```python
from build123d import *

# Parameters (mm, degrees)
F4_DEPTH = 2.3876
F5_SIZE2 = 0.762
F5_SIZE  = 0.762


with BuildPart() as f1:
    # F0 (on Right) → F1 (revolve)
    with BuildSketch(Plane.YZ):
        with BuildLine():
            ThreePointArc((-5.5626, 9.525), (-6.7410456972, 4.8271528886), (-7.1374, 0))
            Line((-7.1374, 0), (7.1374, 0))
            Line((7.1374, 0), (7.1374, 3.175))
            Line((7.1374, 3.175), (-2.3622, 3.175))
            Line((-2.3622, 3.175), (-2.3622, 9.525))
            Line((-2.3622, 9.525), (-5.5626, 9.525))
        make_face()
    revolve(axis=Axis((0, 0, 0), (0, 1, 0)))

    # F3 (on offset) → F4 (cut)
    with BuildSketch(Plane.XZ.offset(7.1374)):
        with BuildLine():
            Line((9.4923983397, 0.7874), (-9.4923983397, 0.7874))
            ThreePointArc((-9.4923983397, 0.7874), (-9.525, 0), (-9.4923983397, -0.7874))
            Line((-9.4923983397, -0.7874), (9.4923983397, -0.7874))
            ThreePointArc((9.4923983397, -0.7874), (9.525, 0), (9.4923983397, 0.7874))
        make_face()
    extrude(amount=-F4_DEPTH, mode=Mode.SUBTRACT)

    # F5
    f5_edges = [f1.edges().sort_by_distance(p)[0] for p in [
        (0, 7.1374, -3.175),
    ]]
    chamfer(f5_edges, length=F5_SIZE, length2=F5_SIZE2)


solid = f1.part
```
Source: CAD feature listing. Evaluate the final solid. Frame: model axes, mm. A direction names the side the tool comes from. Give positions to 0.01 mm unless a question says otherwise; leave off trailing zeros. Write each loop counter-clockwise with the first axis right and the second up, starting at its lowest first coordinate (ties: lowest second). Pieces come first, ordered by that corner, then holes. Notation, with made-up numbers: (69.5, -19.75) - (91.5, -19.75) arc R24 ccw to (91.5, -0.75) - close; hole circle Ø7 at (77, 8.5). An arc over 180 degrees is marked (long way). One line per item, written item: value. Start each with the question number.
Q1. Material intervals for probe 1 along Z at (x, y) = (5.5, -5); probe 2 along Z at (x, y) = (-7.75, -5.5); probe 3 along Y at (x, z) = (-1.75, -0.25), sorted ascending. Write a range as from..to.
Q2. Draft query along Z for faces 1 (the face through (0, 7.137, 0)), 2 (the face through (-5.796, -3.985, -7.559)), 3 (the face through (0, -6, -0.787)). Return one class per face: +Z half, -Z half, draft (parallel to the pull), parting line (faces both ways), or undercut.
Q3. Section query A-A, the plane x = 0. Return the cut outline in (y, z) (3 decimals).
Q4. Set-up query: faces 4 (the face through (0, -4.75, 0)), 5 (the face through (0, -2.362, -4)). Return all of +Z, -Z, +X, -X, +Y, -Y with unobstructed straight access to the full face (end or side cutting, diameter ignored); none if empty.
Q5. Section query B-B, the plane y = -5.25. Return the cut outline in (x, z) (3 decimals), then the cut area to 3 significant figures.
Q6. Section query C-C, the plane z = 0. Return the cut outline in (x, y) (3 decimals), then the cut area to 3 significant figures.
Q7. Section query D-D, the plane y = 2. Return the cut outline in (x, z) (3 decimals), then the cut area to 3 significant figures.
Q8. First-contact query: pin 1 Ø1.5 at (y, z) = (-4.5, 3.5) entering from -X; pin 2 Ø6 at (y, z) = (-3.5, 4) entering from -X; pin 3 Ø8 at (x, z) = (6.5, -7) entering from +Y. Flat tips, straight axial feed; report the tip coordinate or a pass-through.
Answer:
1. probe 1: z = -7.78..-0.79, 0.79..7.78
1. probe 2: z = -5.54..-0.79, 0.79..5.54
1. probe 3: y = -4.75..7.14
2. face 1: draft
2. face 2: parting line
2. face 3: undercut
3. outline: (-7.127, -0.787) arc R29.593 ccw to (-5.563, -9.525) - (-2.362, -9.525) - (-2.362, -3.175) - (6.375, -3.175) - (7.137, -2.413) - (7.137, 2.413) - (6.375, 3.175) - (-2.362, 3.175) - (-2.362, 9.525) - (-5.563, 9.525) arc R29.593 ccw to (-7.127, 0.787) - (-4.75, 0.787) - (-4.75, -0.787) - close
4. face 4: +X, -X, -Y
4. face 5: +Y
5. outline: (-9.492, -0.787) arc R9.525 ccw to (9.492, -0.787) - close; (-9.492, 0.787) - (9.492, 0.787) arc R9.525 ccw to start
5. area: 255 mm2
6. outline: (-9.525, -4.75) - (9.525, -4.75) - (9.525, -2.362) - (3.175, -2.362) - (3.175, 6.375) - (2.413, 7.137) - (-2.413, 7.137) - (-3.175, 6.375) - (-3.175, -2.362) - (-9.525, -2.362) - close
6. area: 105 mm2
7. outline: circle Ø6.35 at (0, 0)
7. area: 31.7 mm2
8. pin 1: stops at x = -9.12
8. pin 2: stops at x = -9.47
8. pin 3: stops at y = -2.36
